Solid Edge part; units mm, degrees
sketch "Sketch1" plane through (0, 0, 0) normal (0, 0, 1) x (1, 0, 0)
  circle A0 centre (0, 0) radius 9
  line L0 (3, 22.5) -> (-3, 22.5)
  arc A1 (-4, 21.5) -> (-3, 22.5) centre (-3, 21.5) cw
  line L1 (-4, 21.5) -> (-4, 14.1421)
  arc A2 (-4.6667, 13.1993) -> (-4, 14.1421) centre (-5, 14.1421) ccw
  arc A3 (-13.7643, -2.5582) -> (-4.6667, 13.1993) centre (0, 0) cw
  arc A4 (-14.2474, -3.607) -> (-13.7643, -2.5582) centre (-14.7474, -2.7409) ccw
  line L2 (-20.6195, -7.2859) -> (-14.2474, -3.607)
  arc A5 (-20.6195, -7.2859) -> (-20.9856, -8.6519) centre (-20.1195, -8.1519) ccw
  line L3 (-17.9856, -13.8481) -> (-20.9856, -8.6519)
  arc A6 (-17.9856, -13.8481) -> (-16.6195, -14.2141) centre (-17.1195, -13.3481) ccw
  line L4 (-10.2474, -10.5352) -> (-16.6195, -14.2141)
  arc A7 (-9.0976, -10.6411) -> (-10.2474, -10.5352) centre (-9.7474, -11.4012) ccw
  arc A8 (10.2474, -10.5352) -> (9.0976, -10.6411) centre (9.7474, -11.4012) ccw
  line L5 (10.2474, -10.5352) -> (16.6195, -14.2141)
  arc A9 (17.9856, -13.8481) -> (16.6195, -14.2141) centre (17.1195, -13.3481) cw
  line L6 (17.9856, -13.8481) -> (20.9856, -8.6519)
  arc A10 (20.6195, -7.2859) -> (20.9856, -8.6519) centre (20.1195, -8.1519) cw
  line L7 (20.6195, -7.2859) -> (14.2474, -3.607)
  arc A11 (13.7643, -2.5582) -> (14.2474, -3.607) centre (14.7474, -2.7409) ccw
  arc A12 (4.6667, 13.1993) -> (13.7643, -2.5582) centre (0, 0) cw
  arc A13 (4, 14.1421) -> (4.6667, 13.1993) centre (5, 14.1421) ccw
  line L8 (4, 14.1421) -> (4, 21.5)
  arc A14 (3, 22.5) -> (4, 21.5) centre (3, 21.5) cw
  arc A15 (-9.0976, -10.6411) -> (9.0976, -10.6411) centre (0, 0) ccw
  circle A16 centre (0, 17.9582) radius 1.5
  circle A17 centre (-15.5523, -8.9791) radius 1.5
  circle A18 centre (15.5523, -8.9791) radius 1.5
extrude "Protrusion1" add sketch "Sketch1" along normal blind 2
Build history of the part. All positions in model axes, mm. A direction names the side the tool comes from. Give positions to 0.01 mm unless a question says otherwise; leave off trailing zeros. Loops run counter-clockwise (first coordinate to the right, second up) from the corner with the lowest first, then second, coordinate; pieces in that order, holes last. Notation, with made-up numbers: (27, -7.5) -> (56, -7.5) arc R15 ccw to (56, 15.5) -> close; hole circle Ø7 at (63, 61.25). An arc over 180 degrees is marked (long way). Answer in a Markdown table with one row per item.
Item 1: Mould opens along X. For faces 1 (the cylindrical face through (13.843, -3.167, 0.986)), 2 (the flat face through (-19.465, -11.286, 0.986)), 3 (the flat face through (-13.39, -12.35, 0.99)), 4 (the cylindrical face through (-1.172, -8.923, 0.986)) say: pulls with the +X half, pulls with the -X half, needs draft (parallel to the pull), parting line crosses it, or undercut.
Findings below:
| item | result |
|---|---|
| face 1 | pulls with the +X half |
| face 2 | pulls with the -X half |
| face 3 | undercut |
| face 4 | undercut |
Item 2: Tool access for faces 5 (the flat face through (13.39, -12.35, 0.99)), 6 (the cylindrical face through (-4.18, 13.57, 0.99)), 7 (the flat face through (4, 18, 1)): list every direction of +Z, -Z, +X, -X, +Y, -Y with a clear straight run to the whole face (end or side of a thin tool).
Findings below:
| item | result |
|---|---|
| face 5 | +Z, -Z, -Y |
| face 6 | +Z, -Z, -X, +Y |
| face 7 | +Z, -Z, +X, +Y |
Item 3: Slice it at C-C on x = -8.5. Write the cut outline in (y, z).
Findings below:
| item | result |
|---|---|
| outline | (-11.12, 0) -> (-2.96, 0) -> (-2.96, 2) -> (-11.12, 2) -> close; (2.96, 0) -> (11.12, 0) -> (11.12, 2) -> (2.96, 2) -> close |
Item 4: Slice it at B-B on y = 0. Write the cut outline in (x, z), plus the area to 3 significant figures.
Findings below:
| item | result |
|---|---|
| outline | (-14, 0) -> (-9, 0) -> (-9, 2) -> (-14, 2) -> close; (9, 0) -> (14, 0) -> (14, 2) -> (9, 2) -> close |
| area | 20.0 mm² |
Item 5: Flat gauge pins, fed straight in: P1, Ø12, axis at x = 9, y = 12, coming from the +Z side; P2, Ø0.6, axis at y = 16, z = 0.5, coming from the -X side. Where does each tip first touch, or does it go through?
Findings below:
| item | result |
|---|---|
| P1 | stops at z = 2 |
| P2 | stops at x = -4 |
Item 6: Slice it at D-D on z = 1.5. Write the cut outline in (x, y).
Findings below:
| item | result |
|---|---|
| outline | (-20.99, -8.65) -> (-17.99, -13.85) arc R1 ccw to (-16.62, -14.21) -> (-10.25, -10.54) arc R1 cw to (-9.1, -10.64) arc R14 ccw to (9.1, -10.64) arc R1 cw to (10.25, -10.54) -> (16.62, -14.21) arc R1 ccw to (17.99, -13.85) -> (20.99, -8.65) arc R1 ccw to (20.62, -7.29) -> (14.25, -3.61) arc R1 cw to (13.76, -2.56) arc R14 ccw to (4.67, 13.2) arc R1 cw to (4, 14.14) -> (4, 21.5) arc R1 ccw to (3, 22.5) -> (-3, 22.5) arc R1 ccw to (-4, 21.5) -> (-4, 14.14) arc R1 cw to (-4.67, 13.2) arc R14 ccw to (-13.76, -2.56) arc R1 cw to (-14.25, -3.61) -> (-20.62, -7.29) arc R1 ccw to start; hole circle Ø3 at (-15.55, -8.98); hole circle Ø18 at (0, 0); hole circle Ø3 at (0, 17.96); hole circle Ø3 at (15.55, -8.98) |
Item 7: Probe line 1 along X through (y, z) = (20, 0.6); line 2 along Y through (x, z) = (-2.5, 1.15); line 3 along X through (y, z) = (17, 0.3). List the from-to ranges inside material, lowest first. Write a range as [from, to].
Findings below:
| item | result |
|---|---|
| line 1 | x = [-4, 4] |
| line 2 | y = [-13.77, -8.65], [8.65, 22.5] |
| line 3 | x = [-4, -1.15], [1.15, 4] |
Item 8: Slice it at A-A on x = 0. Write the cut outline in (y, z), plus the area to 3 significant figures.
Findings below:
| item | result |
|---|---|
| outline | (-14, 0) -> (-9, 0) -> (-9, 2) -> (-14, 2) -> close; (9, 0) -> (16.46, 0) -> (16.46, 2) -> (9, 2) -> close; (19.46, 0) -> (22.5, 0) -> (22.5, 2) -> (19.46, 2) -> close |
| area | 31.0 mm² |
